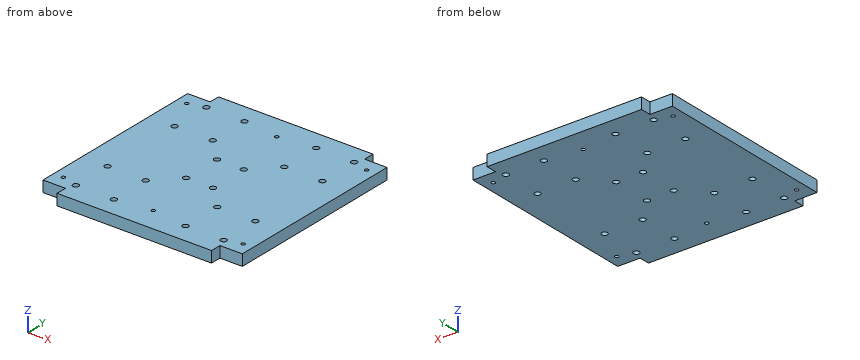
from build123d import *

# Parameters (mm, degrees)
SKETCH1_R           = 2.6
BOSS_EXTRUDE3_DEPTH = 10
M4_TAPPED_HOLE1_D   = 3.3


with BuildPart() as part:
    # Sketch1 → Boss-Extrude3 (new body)
    with BuildSketch(Plane.XY):
        Polygon((-89, 82), (-89, -82), (-69, -82), (-69, -91.5), (69, -91.5), (69, -82), (89, -82), (89, 82), (69, 82), (69, 91.5), (-69, 91.5), (-69, 82), align=None)
        with Locations((-66, 74)):
            Circle(SKETCH1_R, mode=Mode.SUBTRACT)
        with Locations((-32, 74)):
            Circle(SKETCH1_R, mode=Mode.SUBTRACT)
        with Locations((-32, 38)):
            Circle(SKETCH1_R, mode=Mode.SUBTRACT)
        with Locations((-66, 38)):
            Circle(SKETCH1_R, mode=Mode.SUBTRACT)
        with Locations((66, 38)):
            Circle(SKETCH1_R, mode=Mode.SUBTRACT)
        with Locations((32, 38)):
            Circle(SKETCH1_R, mode=Mode.SUBTRACT)
        with Locations((32, 74)):
            Circle(SKETCH1_R, mode=Mode.SUBTRACT)
        with Locations((66, 74)):
            Circle(SKETCH1_R, mode=Mode.SUBTRACT)
        with Locations((66, -74)):
            Circle(SKETCH1_R, mode=Mode.SUBTRACT)
        with Locations((32, -74)):
            Circle(SKETCH1_R, mode=Mode.SUBTRACT)
        with Locations((32, -38)):
            Circle(SKETCH1_R, mode=Mode.SUBTRACT)
        with Locations((66, -38)):
            Circle(SKETCH1_R, mode=Mode.SUBTRACT)
        with Locations((-66, -38)):
            Circle(SKETCH1_R, mode=Mode.SUBTRACT)
        with Locations((-32, -38)):
            Circle(SKETCH1_R, mode=Mode.SUBTRACT)
        with Locations((-32, -74)):
            Circle(SKETCH1_R, mode=Mode.SUBTRACT)
        with Locations((-66, -74)):
            Circle(SKETCH1_R, mode=Mode.SUBTRACT)
        with Locations((-12, 17.5)):
            Circle(SKETCH1_R, mode=Mode.SUBTRACT)
        with Locations((12, 17.5)):
            Circle(SKETCH1_R, mode=Mode.SUBTRACT)
        with Locations((12, -17.5)):
            Circle(SKETCH1_R, mode=Mode.SUBTRACT)
        with Locations((-12, -17.5)):
            Circle(SKETCH1_R, mode=Mode.SUBTRACT)
    extrude(amount=BOSS_EXTRUDE3_DEPTH)

    # M4 Tapped Hole1 (through all)
    with Locations(Plane.XY.offset(10)):
        with Locations((-80.25, 70), (80.25, 70), (0, 70), (0, -70), (80.25, -70), (-80.25, -70)):
            Hole(M4_TAPPED_HOLE1_D / 2)


solid = part.part
Build history of the part. All positions in model axes, mm. Give positions to 0.01 mm unless a question says otherwise; leave off trailing zeros. Order: outer loops, then holes, each group sorted by start corner. A loop starts at its lowest first (then second) coordinate and runs counter-clockwise, first axis right, second up. Notation, with made-up numbers: M 61,23 L 95,23 A18 cw 95,58 Z; hole C 82,71 d2. An arc over 180 degrees is marked long. Put each result on its own line as item: value.
Item 1: Flat gauge pin, fed straight in: pin 1 Ø7 at (x, y) = (-32, 38) entering from -Z. Where does the tip first touch, or does it go through?
From the geometry:
pin 1: stops at z = 0
Item 2: Slice it at C-C, the plane z = 6. Give the number of separate pieces and of enclosed holes in the cut face, plus the area to 3 significant figures.
From the geometry:
separate pieces: 1
enclosed holes: 26
area: 31,300 mm2
Item 3: Slice it at B-B, the plane x = -32. Write the cut outline in (y, z).
From the geometry:
outline: M -91.5,0 L -76.6,0 L -76.6,10 L -91.5,10 Z; M -71.4,0 L -40.6,0 L -40.6,10 L -71.4,10 Z; M -35.4,0 L 35.4,0 L 35.4,10 L -35.4,10 Z; M 40.6,0 L 71.4,0 L 71.4,10 L 40.6,10 Z; M 76.6,0 L 91.5,0 L 91.5,10 L 76.6,10 Z
Item 4: Slice it at A-A, the plane x = -12. Write the cut outline in (y, z).
From the geometry:
outline: M -91.5,0 L -20.1,0 L -20.1,10 L -91.5,10 Z; M -14.9,0 L 14.9,0 L 14.9,10 L -14.9,10 Z; M 20.1,0 L 91.5,0 L 91.5,10 L 20.1,10 Z
Item 5: Probe line 1 (Y direction, x = 32, z = 3); line 2 (Y direction, x = -80.25, z = 2); line 3 (X direction, y = -16.5, z = 2.75). List the from-to ranges inside material, lowest first. Write a range as [from, to].
From the geometry:
line 1: y = [-91.5, -76.6], [-71.4, -40.6], [-35.4, 35.4], [40.6, 71.4], [76.6, 91.5]
line 2: y = [-82, -71.65], [-68.35, 68.35], [71.65, 82]
line 3: x = [-89, -14.4], [-9.6, 9.6], [14.4, 89]
